Read the model definition and answer for the solid it produces. Units are mm, in the model's axes. A direction names the side the tool comes from. Coordinates: 2 decimals unless noted, no trailing zeros. Write each loop counter-clockwise with the first axis right and the second up, starting at its lowest first coordinate (ties: lowest second). Pieces come first, ordered by that corner, then holes.
(1) Find the intervals of material crossed by probe 1 along X at (y, z) = (-5, 8); probe 2 along Y at (x, z) = (13.5, 10.25), in increasing order.
(2) Section A-A on y = 29.5 is taken. Write down the section's boundary in (x, z).
(3) The mould has two halves that part along Y. Classify faces 3 (the flat face through (-2, -76.2, 6)), 4 (the flat face through (152.4, -1, 6)), 5 (the flat face through (104, 50.8, 8)): +Y half, -Y half, draft (parallel to the pull), parting line (faces both ways), or undercut.
(4) Section C-C on x = -109.5 is taken. Write down the section's boundary in (y, z), then the cut area to 3 significant figures.
(5) Given pin 1 (13.5 mm diameter, centred on x = 121.5, y = -13, fed in from +Z), flat-ended and moving along its own axis, determine where the tip first touches the part or whether it passes through.
(6) Which of the six approach directions +Z, -Z, +X, -X, +Y, -Y give full straight-line access (tool end or side, diameter ignored) to faces 1 (the flat face through (-2, 1, 0)), 2 (the flat face through (139.7, 1, 8))?
(7) Section B-B on z = 6.25 is taken. State how many separate pieces and enclosed holes the cut face has, then the cut area to 3 significant figures.
from build123d import *

# Parameters (mm, degrees)
SKETCH1_W           = 304.8
SKETCH1_H           = 152.4
BOSS_EXTRUDE1_DEPTH = 12.7
CUT_EXTRUDE1_DEPTH  = 8.73252
CUT_EXTRUDE2_DEPTH  = 8.73252


with BuildPart() as part:
    # Sketch1 → Boss-Extrude1 (new body)
    with BuildSketch(Plane.XY):
        Rectangle(SKETCH1_W, SKETCH1_H)
    extrude(amount=BOSS_EXTRUDE1_DEPTH)

    # Sketch2 → Cut-Extrude1 (cut)
    with BuildSketch(Plane.XY.offset(12.7)):
        with BuildLine():
            Line((-128.5875, 57.15), (-23.8125, 57.15))
            ThreePointArc((-23.8125, 57.15), (-20.444903955, 55.755096045), (-19.05, 52.3875))
            Line((-19.05, 52.3875), (-19.05, -52.3875))
            ThreePointArc((-19.05, -52.3875), (-20.444903955, -55.755096045), (-23.8125, -57.15))
            Line((-23.8125, -57.15), (-128.5875, -57.15))
            ThreePointArc((-128.5875, -57.15), (-131.955096045, -55.755096045), (-133.35, -52.3875))
            Line((-133.35, -52.3875), (-133.35, 52.3875))
            ThreePointArc((-133.35, 52.3875), (-131.955096045, 55.755096045), (-128.5875, 57.15))
        make_face()
    extrude(amount=-CUT_EXTRUDE1_DEPTH, mode=Mode.SUBTRACT)

    # Sketch3 → Cut-Extrude2 (cut)
    with BuildSketch(Plane.XY.offset(12.7)):
        with BuildLine():
            Line((100.0125, 50.8), (107.95, 50.8))
            Line((107.95, 50.8), (107.95, 58.7375))
            ThreePointArc((107.95, 58.7375), (109.344903955, 62.105096045), (112.7125, 63.5))
            Line((112.7125, 63.5), (134.9375, 63.5))
            ThreePointArc((134.9375, 63.5), (138.305096045, 62.105096045), (139.7, 58.7375))
            Line((139.7, 58.7375), (139.7, 50.8))
            Line((139.7, 50.8), (139.7, -58.7375))
            ThreePointArc((139.7, -58.7375), (138.305096045, -62.105096045), (134.9375, -63.5))
            Line((134.9375, -63.5), (100.0125, -63.5))
            ThreePointArc((100.0125, -63.5), (96.644903955, -62.105096045), (95.25, -58.7375))
            Line((95.25, -58.7375), (95.25, 46.0375))
            ThreePointArc((95.25, 46.0375), (96.644903955, 49.405096045), (100.0125, 50.8))
        make_face()
        with BuildLine():
            Line((11.1125, 63.5), (65.0875, 63.5))
            ThreePointArc((65.0875, 63.5), (68.455096045, 62.105096045), (69.85, 58.7375))
            Line((69.85, 58.7375), (69.85, -58.7375))
            ThreePointArc((69.85, -58.7375), (68.455096045, -62.105096045), (65.0875, -63.5))
            Line((65.0875, -63.5), (11.1125, -63.5))
            ThreePointArc((11.1125, -63.5), (7.744903955, -62.105096045), (6.35, -58.7375))
            Line((6.35, -58.7375), (6.35, 58.7375))
            ThreePointArc((6.35, 58.7375), (7.744903955, 62.105096045), (11.1125, 63.5))
        make_face()
    extrude(amount=-CUT_EXTRUDE2_DEPTH, mode=Mode.SUBTRACT)


solid = part.part
Response:
1. probe 1: x = -152.4 to -133.35, -19.05 to 6.35, 69.85 to 95.25, 139.7 to 152.4
1. probe 2: y = -76.2 to -63.5, 63.5 to 76.2
2. outline: (-152.4, 0) - (152.4, 0) - (152.4, 12.7) - (139.7, 12.7) - (139.7, 3.97) - (95.25, 3.97) - (95.25, 12.7) - (69.85, 12.7) - (69.85, 3.97) - (6.35, 3.97) - (6.35, 12.7) - (-19.05, 12.7) - (-19.05, 3.97) - (-133.35, 3.97) - (-133.35, 12.7) - (-152.4, 12.7) - close
3. face 3: -Y half
3. face 4: draft
3. face 5: undercut
4. outline: (-76.2, 0) - (76.2, 0) - (76.2, 12.7) - (57.15, 12.7) - (57.15, 3.97) - (-57.15, 3.97) - (-57.15, 12.7) - (-76.2, 12.7) - close
4. area: 937 mm2
5. pin 1: stops at z = 3.97
6. face 1: -Z, +X, -X, +Y, -Y
6. face 2: +Z
7. separate pieces: 1
7. enclosed holes: 3
7. area: 19,900 mm2
